Source: CAD feature listing. Evaluate the final solid. Frame: model axes, mm. Face numbers are marked on the shaded views. A direction names the side the tool comes from. Coordinates: 2 decimals unless noted, no trailing zeros. Order: outer loops, then holes, each group sorted by start corner. A loop starts at its lowest first (then second) coordinate and runs counter-clockwise, first axis right, second up. Notation, with made-up numbers: (-39, 33.25) -> (-29, 33.25) arc R24 ccw to (-29, 46.25) -> close; hole circle Ø9 at (75, -11). An arc over 180 degrees is marked (long way). Put each result on its own line as item: value.
from build123d import *

# Parameters (mm, degrees)
SALIENTE_EXTRUIR1_DEPTH = 30
CORTAR_EXTRUIR1_DEPTH   = 3.5
CORTAR_EXTRUIR2_DEPTH   = 46.219685979
CROQUIS4_W              = 10
CROQUIS4_H              = 1.5
CORTAR_EXTRUIR3_DEPTH   = 3.5
CROQUIS5_W              = 35.3
CROQUIS5_H              = 10.3
SALIENTE_EXTRUIR2_DEPTH = 2


with BuildPart() as part:
    # Croquis1 → Saliente-Extruir1 (new body)
    with BuildSketch(Plane.XY):
        Polygon((0, 0), (30.5, 0), (30.5, 2), (29.5, 2), (29.5, 4.4), (32.9, 4.4), (32.9, -5.9), (-2.4, -5.9), (-2.4, 4.4), (1, 4.4), (1, 2), (0, 2), align=None)
    extrude(amount=SALIENTE_EXTRUIR1_DEPTH)

    # Croquis2 → Cortar-Extruir1 (cut)
    with BuildSketch(Plane(origin=(0, 0, 0), x_dir=(1, 0, 0), z_dir=(0, 1, 0))):
        with BuildLine():
            Line((5, -15), (5, 0))
            Line((5, 0), (25.5, 0))
            Line((25.5, 0), (25.5, -15))
            ThreePointArc((25.5, -15), (15.25, -25.25), (5, -15))
        make_face()
    extrude(amount=-CORTAR_EXTRUIR1_DEPTH, mode=Mode.SUBTRACT)

    # Croquis3 → Cortar-Extruir2 (cut, through all)
    with BuildSketch(Plane(origin=(0, -3.5, 0), x_dir=(1, 0, 0), z_dir=(0, 1, 0))):
        with BuildLine():
            Line((10.25, -20.25), (10.25, 0))
            Line((10.25, 0), (20.25, 0))
            Line((20.25, 0), (20.25, -20.25))
            ThreePointArc((20.25, -20.25), (15.25, -25.25), (10.25, -20.25))
        make_face()
    extrude(amount=-CORTAR_EXTRUIR2_DEPTH, mode=Mode.SUBTRACT)

    # Croquis4 → Cortar-Extruir3 (cut)
    with BuildSketch(Plane.ZY.offset(-30.5)):
        with Locations((15, 0.75)):
            Rectangle(CROQUIS4_W, CROQUIS4_H)
    extrude(amount=-CORTAR_EXTRUIR3_DEPTH, mode=Mode.SUBTRACT)

    # Croquis5 → Saliente-Extruir2 (add)
    with BuildSketch(Plane.XY.offset(30)):
        with Locations((15.25, -0.75)):
            Rectangle(CROQUIS5_W, CROQUIS5_H)
    extrude(amount=SALIENTE_EXTRUIR2_DEPTH)


solid = part.part
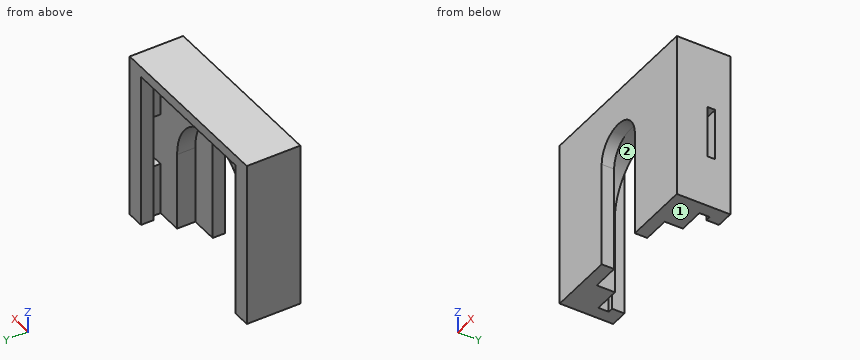
1. Cut plane C-C on z = 24.5. Output: boundary loops of the cut face in (x, y).
Numbers:
outline: (-2.4, -5.9) -> (12.62, -5.9) -> (12.62, -3.5) -> (11.4, -3.5) -> (11.4, 0) -> (0, 0) -> (0, 2) -> (1, 2) -> (1, 4.4) -> (-2.4, 4.4) -> close; (17.88, -5.9) -> (32.9, -5.9) -> (32.9, 4.4) -> (29.5, 4.4) -> (29.5, 2) -> (30.5, 2) -> (30.5, 0) -> (19.1, 0) -> (19.1, -3.5) -> (17.88, -3.5) -> close
2. Set-up query: the marked faces 1 and 2. Return all of +Z, -Z, +X, -X, +Y, -Y with unobstructed straight access to the full face (end or side cutting, diameter ignored); none if empty.
Numbers:
face 1: -Z, +X, -X, +Y, -Y
face 2: -Z, +Y
3. Cut plane B-B on y = -4.75. Output: boundary loops of the cut face in (x, z), plus the area to 3 significant figures.
Numbers:
outline: (-2.4, 0) -> (10.25, 0) -> (10.25, 20.25) arc R5 cw to (20.25, 20.25) -> (20.25, 0) -> (32.9, 0) -> (32.9, 32) -> (-2.4, 32) -> close
area: 888 mm2
4. Cut plane A-A on z = 10.5. Output: boundary loops of the cut face in (x, y), plus the area to 3 significant figures.
Numbers:
outline: (-2.4, -5.9) -> (10.25, -5.9) -> (10.25, -3.5) -> (5, -3.5) -> (5, 0) -> (0, 0) -> (0, 2) -> (1, 2) -> (1, 4.4) -> (-2.4, 4.4) -> close; (20.25, -5.9) -> (32.9, -5.9) -> (32.9, 0) -> (25.5, 0) -> (25.5, -3.5) -> (20.25, -3.5) -> close; (29.5, 2) -> (30.5, 2) -> (30.5, 1.5) -> (32.9, 1.5) -> (32.9, 4.4) -> (29.5, 4.4) -> close
area: 135 mm2
5. First-contact query: pin 1 (8 mm diameter, centred on x = 11, z = 6.5, fed in from +Y); pin 2 (1.5 mm diameter, centred on x = 2.5, z = 12, fed in from +Y); pin 3 (0.6 mm diameter, centred on y = 1, z = 14.5, fed in from +X). Flat tips, straight axial feed; report the tip coordinate or a pass-through.
Numbers:
pin 1: stops at y = -3.5
pin 2: stops at y = 0
pin 3: stops at x = 0
6. Cut plane D-D on x = 26.5. Output: boundary loops of the cut face in (y, z).
Numbers:
outline: (-5.9, 0) -> (0, 0) -> (0, 30) -> (4.4, 30) -> (4.4, 32) -> (-5.9, 32) -> close
7. Ray query, line 1 along X through (y, z) = (2.5, 14.5); line 2 along X through (y, z) = (-2.5, 11.5); line 3 along Y through (x, z) = (28, 2). Return the intervals inside material, ascending.
Numbers:
line 1: x = -2.4 to 1, 29.5 to 32.9
line 2: x = -2.4 to 5, 25.5 to 32.9
line 3: y = -5.9 to 0
